from build123d import *

# Parameters (mm, degrees)
SKETCH3_R          = 0.875
CUT_EXTRUDE1_DEPTH = 2
CHAMFER1_SIZE      = 0.5
FILLET1_R          = 0.2
FILLET2_R          = 0.2


with BuildPart() as part:
    # Sketch2 → Revolve1 (revolve)
    with BuildSketch(Plane.XY):
        Polygon((0, 2), (0, 4.5), (2, 4.5), (2, 1.5), (3.5, 1.5), (3.5, 0), (1.2, 0), (1.2, 2), align=None)
    revolve(axis=Axis((0, 2, 0), (0, 1, 0)))

    # Sketch3 → Cut-Extrude1 (cut)
    with BuildSketch(Plane(origin=(0, 4.5, 0), x_dir=(1, 0, 0), z_dir=(0, 1, 0))):
        Circle(SKETCH3_R)
    extrude(amount=-CUT_EXTRUDE1_DEPTH, mode=Mode.SUBTRACT)

    # Chamfer1
    chamfer1_edges = [part.edges().sort_by_distance(p)[0] for p in [
        (-2, 4.5, 0),
    ]]
    chamfer(chamfer1_edges, length=CHAMFER1_SIZE)

    # Fillet1
    fillet1_edges = [part.edges().sort_by_distance(p)[0] for p in [
        (-2, 1.5, 0),
    ]]
    fillet(fillet1_edges, radius=FILLET1_R)

    # Fillet2
    fillet2_edges = [part.edges().sort_by_distance(p)[0] for p in [
        (-0.875, 2.5, 0),
        (-1.2, 2, 0),
    ]]
    fillet(fillet2_edges, radius=FILLET2_R)


solid = part.part
Read the model definition and answer for the solid it produces. Units are mm, in the model's axes. A direction names the side the tool comes from. Coordinates: 2 decimals unless noted, no trailing zeros. Write each loop counter-clockwise with the first axis right and the second up, starting at its lowest first coordinate (ties: lowest second). Pieces come first, ordered by that corner, then holes. Notation, with made-up numbers: M -40,23.25 L -5,23.25 A31 ccw -5,57.25 Z; hole C 30,-17 d10. An arc over 180 degrees is marked long. Use a Markdown table: item, result.
Q1. The part is cut by section D-D, the plane y = 3.2. Write down the section's boundary in (x, z) (3 decimals).
Answer block:
| item | result |
|---|---|
| outline | C 0,0 d4; hole C 0,0 d1.75 |
Q2. The part is cut by section C-C, the plane y = 1.1. Write down the section's boundary in (x, z).
Answer block:
| item | result |
|---|---|
| outline | C 0,0 d7; hole C 0,0 d2.4 |
Q3. Determine the mould class of faces 1 (the face through (3.233, 0.74, 1.341)), 2 (the face through (0, 2, 0)), 3 (the face through (2, 1.5, 2)) for opening direction X: released by +X, released by -X, zero draft, split by the parting line, or undercut.
Answer block:
| item | result |
|---|---|
| face 1 | split by the parting line |
| face 2 | undercut |
| face 3 | zero draft |
Q4. The part is cut by section A-A, the plane z = 0. Write down the section's boundary in (x, y) (3 decimals), then the cut area to 3 significant figures.
Answer block:
| item | result |
|---|---|
| outline | M -3.5,0 L -1.2,0 L -1.2,1.8 A0.2 cw -1,2 L 1,2 A0.2 cw 1.2,1.8 L 1.2,0 L 3.5,0 L 3.5,1.5 L 2.2,1.5 A0.2 cw 2,1.7 L 2,4 L 1.5,4.5 L 0.875,4.5 L 0.875,2.7 A0.2 cw 0.675,2.5 L -0.675,2.5 A0.2 cw -0.875,2.7 L -0.875,4.5 L -1.5,4.5 L -2,4 L -2,1.7 A0.2 cw -2.2,1.5 L -3.5,1.5 Z |
| area | 14.0 mm2 |
Q5. Straight lines are drawn through the part: L1, parallel to X at y = 3.55, z = 0 (3 decimals); L2, parallel to Z at x = 0, y = 0.4. For each, find the intervals that lie inside material, in ascending order. Write a range as [from, to].
Answer block:
| item | result |
|---|---|
| L1 | x = [-2, -0.875], [0.875, 2] |
| L2 | z = [-3.5, -1.2], [1.2, 3.5] |
Q6. Which of the six approach directions +Z, -Z, +X, -X, +Y, -Y give full straight-line access (tool end or side, diameter ignored) to faces 4 (the face through (0, 3, 2)), 5 (the face through (0.65, 0.91, -1.01)), 6 (the face through (0, 0, 2))?
Answer block:
| item | result |
|---|---|
| face 4 | +Y |
| face 5 | -Y |
| face 6 | +Z, -Z, +X, -X, -Y |
Q7. Each of these flat-tipped pins is pushed along its axis until it touches: pin 1 Ø1 at (x, y) = (-1, 1.5) entering from -Z; pin 2 Ø1 at (x, y) = (2, 3.5) entering from +Z; pin 3 Ø2 at (x, z) = (0, 0) entering from -Y. Where does it stop, or does it pass through?
Answer block:
| item | result |
|---|---|
| pin 1 | stops at z = -3.46 |
| pin 2 | stops at z = 1.32 |
| pin 3 | stops at y = 2 |
Q8. The part is cut by section B-B, the plane x = 0. Write down the section's boundary in (y, z) (3 decimals).
Answer block:
| item | result |
|---|---|
| outline | M 0,-3.5 L 1.5,-3.5 L 1.5,-2.2 A0.2 cw 1.7,-2 L 4,-2 L 4.5,-1.5 L 4.5,-0.875 L 2.7,-0.875 A0.2 cw 2.5,-0.675 L 2.5,0.675 A0.2 cw 2.7,0.875 L 4.5,0.875 L 4.5,1.5 L 4,2 L 1.7,2 A0.2 cw 1.5,2.2 L 1.5,3.5 L 0,3.5 L 0,1.2 L 1.8,1.2 A0.2 cw 2,1 L 2,-1 A0.2 cw 1.8,-1.2 L 0,-1.2 Z |
